Build history of the part. All positions in model axes, mm. A direction names the side the tool comes from. Coordinates: 2 decimals unless noted, no trailing zeros. Loops run counter-clockwise (first coordinate to the right, second up) from the corner with the lowest first, then second, coordinate; pieces in that order, holes last.
(1) Slice it at D-D (z = -39). Give the cut face in (x, y), and give its area (3 significant figures).
(2) Two-plate mould, pull along X, no slides. Class faces 6 (the face through (12.07, -31.21, -66.82)), 7 (the face through (26, 0, -33)), 8 (the face through (6.459, 1.288, -21.537)): pulls with the +X half, pulls with the -X half, needs draft (parallel to the pull), parting line crosses it, or undercut.
(3) Slice it at A-A (z = -19.05). Give the cut face in (x, y).
(4) Slice it at C-C (x = 20). Give the cut face in (y, z), and give its area (3 significant figures).
(5) Tool access for faces 1 (the face through (6.459, 1.288, -34.237)), 2 (the face through (49.53, -12, -67)), 3 (the face through (1.81, 1.29, -1.91)), 4 (the face through (10.16, -12, -67)), 5 (the face through (30, -17, -65.532)): list every direction of +Z, -Z, +X, -X, +Y, -Y with a clear straight run to the whole face (end or side of a thin tool).
(6) Wall check: L1, parallel to X at y = 2, z = -19.05; L2, parallel to X at y = -20.32, z = -67.35; L3, parallel to Z at x = 45.5, y = -21.5. Give the ranges that are in metal, low to high.
(7) Flat gauge pins, fed straight in: P1, Ø5, axis at y = -3.5, z = -20.5, coming from the +X side; P2, Ø1, axis at x = 41.5, y = -13.5, coming from the +Z side; P3, Ø1.7, axis at y = -19, z = -66.5, coming from the -X side; P4, Ø1.5, axis at x = 34, z = -12.5, coming from the -Y side. Where does each tip first touch, or does it go through?
(8) Slice it at B-B (x = 5). Give the cut face in (y, z).
from build123d import *

# Parameters (mm, degrees)
SKETCH1_R           = 2.4892
SKETCH1_R_2         = 1.4224
BOSS_EXTRUDE1_DEPTH = 3.175
BASE_FLANGE1_DEPTH  = 2.54
EDGE_FLANGE1_START  = 10.16
EDGE_FLANGE1_DEPTH  = 39.37
SKETCH10_R          = 2.4892
CUT_EXTRUDE1_DEPTH  = 115.617842028
SKETCH11_R          = 1.4224
CUT_EXTRUDE2_DEPTH  = 93.32708809
FILLET1_R           = 6.35


# Read off the part's stored shape, not the designer's step: Edge-Flange1
# Sheet-metal steps are written as plain solids
with BuildPart() as part:
    # Sketch1 → Boss-Extrude1 (new body)
    with BuildSketch(Plane(origin=(0, 0, 0), x_dir=(1, 0, 0), z_dir=(0, 1, 0))):
        Polygon((0, 0), (52.916666667, 0), (52.916666667, 44.45), (44.45, 95.25), (25.4, 95.25), (0, 44.45), align=None)
        with Locations(Location((6.35, 6.35, 0), (0, 0, 270))):
            Circle(SKETCH1_R, mode=Mode.SUBTRACT)
        with Locations(Location((6.35, 19.05, 0), (0, 0, 270))):
            Circle(SKETCH1_R, mode=Mode.SUBTRACT)
        with Locations(Location((6.35, 31.75, 0), (0, 0, 270))):
            Circle(SKETCH1_R, mode=Mode.SUBTRACT)
        with Locations(Location((46.566666667, 6.35, 0), (0, 0, 270))):
            Circle(SKETCH1_R, mode=Mode.SUBTRACT)
        with Locations(Location((46.566666667, 19.05, 0), (0, 0, 270))):
            Circle(SKETCH1_R, mode=Mode.SUBTRACT)
        with Locations(Location((46.566666667, 31.75, 0), (0, 0, 270))):
            Circle(SKETCH1_R, mode=Mode.SUBTRACT)
        with Locations(Location((31.75508, 82.56016, 0), (0, 0, 270))):
            Circle(SKETCH1_R_2, mode=Mode.SUBTRACT)
        with Locations(Location((39.755080002, 82.56016, 0), (0, 0, 270))):
            Circle(SKETCH1_R_2, mode=Mode.SUBTRACT)
    extrude(amount=BOSS_EXTRUDE1_DEPTH)


with BuildPart() as body_2:
    # Sketch2 → Base-Flange1 (new body)
    with BuildSketch(Plane(origin=(0, 0, 0), x_dir=(1, 0, 0), z_dir=(0, 1, 0))):
        Polygon((0, 0), (52.916666667, 0), (52.916666667, 44.45), (49.53, 64.77), (10.16, 64.77), (0, 44.45), align=None)
    extrude(amount=BASE_FLANGE1_DEPTH)

    # Edge-Flange1 outline → Edge-Flange1 (add)
    with BuildSketch(Plane.YZ.offset(EDGE_FLANGE1_START)):
        with BuildLine():
            Line((-33.02, -68.072), (-0.762, -68.072))
            ThreePointArc((-0.762, -68.072), (1.572866591, -67.104866591), (2.54, -64.77))
            Line((2.54, -64.77), (0, -64.77))
            ThreePointArc((0, -64.77), (-0.223184633, -65.308815367), (-0.762, -65.532))
            Line((-0.762, -65.532), (-33.02, -65.532))
            Line((-33.02, -65.532), (-33.02, -68.072))
        make_face()
    extrude(amount=EDGE_FLANGE1_DEPTH)

    # Sketch10 → Cut-Extrude1 (cut, through all)
    with BuildSketch(Plane(origin=(0, 2.54, 0), x_dir=(1, 0, 0), z_dir=(0, 1, 0))):
        with Locations(Location((46.566666667, 31.75, 0), (0, 0, 270))):
            Circle(SKETCH10_R)
        with Locations(Location((46.566666667, 19.05, 0), (0, 0, 270))):
            Circle(SKETCH10_R)
        with Locations(Location((46.566666667, 6.35, 0), (0, 0, 270))):
            Circle(SKETCH10_R)
        with Locations(Location((6.35, 6.35, 0), (0, 0, 270))):
            Circle(SKETCH10_R)
        with Locations(Location((6.35, 19.05, 0), (0, 0, 270))):
            Circle(SKETCH10_R)
        with Locations(Location((6.35, 31.75, 0), (0, 0, 270))):
            Circle(SKETCH10_R)
    extrude(amount=-CUT_EXTRUDE1_DEPTH, mode=Mode.SUBTRACT)

    # Sketch11 → Cut-Extrude2 (cut, through all)
    with BuildSketch(Plane(origin=(0, 0, -68.072), x_dir=(-1, 0, 0), z_dir=(0, 0, -1))):
        with Locations(Location((-34.035000002, -20.32, 0), (0, 0, 90))):
            Circle(SKETCH11_R)
        with Locations(Location((-26.035, -20.32, 0), (0, 0, 90))):
            Circle(SKETCH11_R)
    extrude(amount=-CUT_EXTRUDE2_DEPTH, mode=Mode.SUBTRACT)

    # Fillet1
    fillet1_edges = [body_2.edges().sort_by_distance(p)[0] for p in [
        (0, 1.27, -44.45),
        (52.916666667, 1.27, -44.45),
        (52.916666667, 1.27, 0),
        (0, 1.27, 0),
        (10.16, -33.02, -66.802),
        (49.53, -33.02, -66.802),
    ]]
    fillet(fillet1_edges, radius=FILLET1_R)


solid = body_2.part
Response values:
1. outline: (0, 0) - (52.92, 0) - (52.92, 2.54) - (0, 2.54) - close
1. area: 134 mm2
2. face 6: pulls with the -X half
2. face 7: needs draft
2. face 8: undercut
3. outline: (0, 0) - (3.86, 0) - (3.86, 2.54) - (0, 2.54) - close; (8.84, 0) - (44.08, 0) - (44.08, 2.54) - (8.84, 2.54) - close; (49.06, 0) - (52.92, 0) - (52.92, 2.54) - (49.06, 2.54) - close
4. outline: (-33.02, -68.07) - (-0.76, -68.07) arc R3.3 ccw to (2.54, -64.77) - (2.54, 0) - (0, 0) - (0, -64.77) arc R0.76 cw to (-0.76, -65.53) - (-33.02, -65.53) - close
4. area: 255 mm2
5. face 1: +Y, -Y
5. face 2: -Z, +X, +Y, -Y
5. face 3: +Z, -X, +Y, -Y
5. face 4: -Z, -X, +Y, -Y
5. face 5: +Z, +X, -X, -Y
6. L1: x = 0 to 3.86, 8.84 to 44.08, 49.06 to 52.92
6. L2: x = 10.16 to 24.61, 27.46 to 32.61, 35.46 to 49.53
6. L3: z = -68.07 to -65.53
7. P1: passes through
7. P2: stops at z = -65.53
7. P3: stops at x = 10.16
7. P4: stops at y = 0
8. outline: (0, -54.45) - (2.54, -54.45) - (2.54, -33.84) - (0, -33.84) - close; (0, -29.66) - (2.54, -29.66) - (2.54, -21.14) - (0, -21.14) - close; (0, -16.96) - (2.54, -16.96) - (2.54, -8.44) - (0, -8.44) - close; (0, -4.26) - (2.54, -4.26) - (2.54, -0.15) - (0, -0.15) - close
